from build123d import *

# Parameters (mm, degrees)
ESQUISSE2_W             = 165
ESQUISSE2_H             = 165
BASE_DEPTH              = 30
ESQUISSE3_R             = 15
BLOC_MOTEUR_1_DEPTH     = 80
ESQUISSE4_W             = 10
ESQUISSE4_H             = 22.360679774
ACCES_MOTEUR_DEPTH      = 37
ESQUISSE6_R             = 16.01
BLOC_MOTEUR_2_DEPTH     = 37
ESQUISSE7_R             = 2.5
VIS_MOTEUR_DEPTH        = 121.467838032
ESQUISSE8_R             = 2.5
VIS_PATIN_DEPTH         = 121.467838032
ESQUISSE12_R            = 30
ESPACE_ROUE_DEPTH       = 10
FIXE_PORTE_1_DEPTH      = 2.5
FIXE_PORTE_1_DEPTH_BACK = 10
ESQUISSE14_R            = 2
ESQUISSE15_W            = 5
ESQUISSE15_H            = 10.139320225
FIXE_PORTE_2_DEPTH      = 2.5
ESQUISSE16_R            = 2
FIXE_PORTE_3_DEPTH      = 10
ESQUISSE18_R            = 2
VIDE_CORDE_COTE_DEPTH   = 75
ESQUISSE19_R            = 2
VIDEO_CORDE_HAUT_DEPTH  = 5
CONGE_CORDE_R           = 0.8
ESQUISSE20_R            = 2
BOSS_MAX_PORTE_DEPTH    = 2
ESQUISSE23_W            = 10
ESQUISSE23_H            = 30
VIDE_TIGE_DEPTH         = 10
VIDE_VIS_REACH          = 185.737
ESQUISSE25_R            = 2.5


with BuildPart() as part:
    # Esquisse2 → BASE (new body)
    with BuildSketch(Plane(origin=(0, 0, 0), x_dir=(1, 0, 0), z_dir=(0, 1, 0))):
        Rectangle(ESQUISSE2_W, ESQUISSE2_H)
    extrude(amount=BASE_DEPTH)

    # Esquisse3 → BLOC MOTEUR 1. (cut)
    with BuildSketch(Plane(origin=(82.5, 0, 0), x_dir=(0, 0, -1), z_dir=(1, 0, 0))):
        with Locations((50, 10)):
            Circle(ESQUISSE3_R)
    bloc_moteur_1 = extrude(amount=-BLOC_MOTEUR_1_DEPTH, mode=Mode.SUBTRACT)

    # Esquisse4 → ACCES MOTEUR (cut)
    with BuildSketch(Plane.XZ):
        with Locations((7.5, -50)):
            Rectangle(ESQUISSE4_W, ESQUISSE4_H)
    acces_moteur = extrude(amount=-ACCES_MOTEUR_DEPTH, mode=Mode.SUBTRACT)

    # Esquisse6 → BLOC MOTEUR 2 (cut)
    with BuildSketch(Plane(origin=(82.5, 0, 0), x_dir=(0, 0, -1), z_dir=(1, 0, 0))):
        with Locations((50, 10)):
            Circle(ESQUISSE6_R)
    bloc_moteur_2 = extrude(amount=-BLOC_MOTEUR_2_DEPTH, mode=Mode.SUBTRACT)

    # SYM BLOC MOTEUR: BLOC MOTEUR 1., ACCES MOTEUR, BLOC MOTEUR 2 across plane
    add(bloc_moteur_1.mirror(Plane(origin=(0, 0, 0), x_dir=(0, 0, 1), z_dir=(1, 0, 0))), mode=Mode.SUBTRACT)
    add(acces_moteur.mirror(Plane(origin=(0, 0, 0), x_dir=(0, 0, 1), z_dir=(1, 0, 0))), mode=Mode.SUBTRACT)
    add(bloc_moteur_2.mirror(Plane(origin=(0, 0, 0), x_dir=(0, 0, 1), z_dir=(1, 0, 0))), mode=Mode.SUBTRACT)

    # Esquisse7 → VIS MOTEUR (cut, through all)
    with BuildSketch(Plane.XZ):
        with Locations(Location((-64, -27.497196314, 0), (0, 0, 270))):
            Circle(ESQUISSE7_R)
        with Locations(Location((-24, -28.819660113, 0), (0, 0, 270))):
            Circle(ESQUISSE7_R)
        with Locations(Location((-24, -71.180339887, 0), (0, 0, 270))):
            Circle(ESQUISSE7_R)
        with Locations(Location((-64, -72.502803686, 0), (0, 0, 270))):
            Circle(ESQUISSE7_R)
    vis_moteur = extrude(amount=-VIS_MOTEUR_DEPTH, mode=Mode.SUBTRACT)

    # SYM VIS: VIS MOTEUR across plane
    add(vis_moteur.mirror(Plane(origin=(0, 0, 0), x_dir=(0, 0, 1), z_dir=(1, 0, 0))), mode=Mode.SUBTRACT)

    # Esquisse8 → VIS PATIN (cut, through all)
    with BuildSketch(Plane.XZ):
        with Locations(Location((-52.5, 52.5, 0), (0, 0, 270))):
            Circle(ESQUISSE8_R)
        with Locations(Location((52.5, 52.5, 0), (0, 0, 270))):
            Circle(ESQUISSE8_R)
    extrude(amount=-VIS_PATIN_DEPTH, mode=Mode.SUBTRACT)

    # Esquisse12 → ESPACE ROUE (cut)
    with BuildSketch(Plane.ZY.offset(82.5)):
        with Locations((-50, 10)):
            Circle(ESQUISSE12_R)
    espace_roue = extrude(amount=-ESPACE_ROUE_DEPTH, mode=Mode.SUBTRACT)

    # SYM ESPACE ROUE: ESPACE ROUE across plane
    add(espace_roue.mirror(Plane(origin=(0, 0, 0), x_dir=(0, 0, 1), z_dir=(1, 0, 0))), mode=Mode.SUBTRACT)

    # Esquisse14 → FIXE PORTE 1 (add, two sides: drawn at the far end of the back side and taken through both)
    # profile 1 of 2: a face of its own
    with BuildSketch(Plane(origin=(0, 30, 0), x_dir=(1, 0, 0), z_dir=(0, 1, 0)).offset(-FIXE_PORTE_1_DEPTH_BACK)):
        with BuildLine():
            ThreePointArc((-77.5, 87.245138583), (-80, 89.745138583), (-82.5, 87.245138583))
            Line((-82.5, 87.245138583), (-82.5, 82.5))
            Line((-82.5, 82.5), (-77.5, 82.5))
            Line((-77.5, 82.5), (-77.5, 87.245138583))
        make_face()
        with Locations(Location((-80, 87.245138583, 0), (0, 0, 270))):
            Circle(ESQUISSE14_R, mode=Mode.SUBTRACT)
    # profile 2 of 2: a face of its own
    with BuildSketch(Plane(origin=(0, 30, 0), x_dir=(1, 0, 0), z_dir=(0, 1, 0)).offset(-FIXE_PORTE_1_DEPTH_BACK)):
        with BuildLine():
            Line((77.5, 87.245138583), (77.5, 82.5))
            Line((77.5, 82.5), (82.5, 82.5))
            Line((82.5, 82.5), (82.5, 87.245138583))
            ThreePointArc((82.5, 87.245138583), (80, 89.745138583), (77.5, 87.245138583))
        make_face()
        with Locations(Location((80, 87.245138583, 0), (0, 0, 270))):
            Circle(ESQUISSE14_R, mode=Mode.SUBTRACT)
    extrude(amount=FIXE_PORTE_1_DEPTH + FIXE_PORTE_1_DEPTH_BACK)

    # Esquisse15 → FIXE PORTE 2 (add)
    with BuildSketch(Plane(origin=(0, 30, 0), x_dir=(1, 0, 0), z_dir=(0, 1, 0))):
        with Locations((-80, 77.430339887)):
            Rectangle(ESQUISSE15_W, ESQUISSE15_H)
        with Locations((80, 77.430339887)):
            Rectangle(ESQUISSE15_W, ESQUISSE15_H)
    extrude(amount=FIXE_PORTE_2_DEPTH)

    # Esquisse16 → FIXE PORTE 3 (add)
    # profile 1 of 2: a face of its own
    with BuildSketch(Plane.XZ):
        with BuildLine():
            Line((-82.5, -82.5), (-82.5, -87.245138583))
            ThreePointArc((-82.5, -87.245138583), (-80, -89.745138583), (-77.5, -87.245138583))
            Line((-77.5, -87.245138583), (-77.5, -82.5))
            Line((-77.5, -82.5), (-82.5, -82.5))
        make_face()
        with Locations(Location((-80, -87.245138583, 0), (0, 0, 90))):
            Circle(ESQUISSE16_R, mode=Mode.SUBTRACT)
    # profile 2 of 2: a face of its own
    with BuildSketch(Plane.XZ):
        with BuildLine():
            Line((82.5, -82.5), (77.5, -82.5))
            Line((77.5, -82.5), (77.5, -87.245138583))
            ThreePointArc((77.5, -87.245138583), (80, -89.745138583), (82.5, -87.245138583))
            Line((82.5, -87.245138583), (82.5, -82.5))
        make_face()
        with Locations(Location((80, -87.245138583, 0), (0, 0, 90))):
            Circle(ESQUISSE16_R, mode=Mode.SUBTRACT)
    extrude(amount=-FIXE_PORTE_3_DEPTH)

    # Esquisse18 → VIDE CORDE COTE (cut)
    with BuildSketch(Plane(origin=(82.5, 0, 0), x_dir=(0, 0, -1), z_dir=(1, 0, 0))):
        with Locations((79.5, 27)):
            Circle(ESQUISSE18_R)
    vide_corde_cote = extrude(amount=-VIDE_CORDE_COTE_DEPTH, mode=Mode.SUBTRACT)

    # Esquisse19 → VIDEO CORDE HAUT (cut)
    with BuildSketch(Plane(origin=(0, 30, 0), x_dir=(1, 0, 0), z_dir=(0, 1, 0))):
        with Locations(Location((9.5, 79.5, 0), (0, 0, 270))):
            Circle(ESQUISSE19_R)
    video_corde_haut = extrude(amount=-VIDEO_CORDE_HAUT_DEPTH, mode=Mode.SUBTRACT)

    # SYM CORDE: VIDE CORDE COTE, VIDEO CORDE HAUT across plane
    add(vide_corde_cote.mirror(Plane(origin=(0, 0, 0), x_dir=(0, 0, 1), z_dir=(1, 0, 0))), mode=Mode.SUBTRACT)
    add(video_corde_haut.mirror(Plane(origin=(0, 0, 0), x_dir=(0, 0, 1), z_dir=(1, 0, 0))), mode=Mode.SUBTRACT)

    # CONGE CORDE
    conge_corde_edges = [part.edges().sort_by_distance(p)[0] for p in [
        (9.5, 30, -81.5),
        (-9.5, 30, -81.5),
    ]]
    fillet(conge_corde_edges, radius=CONGE_CORDE_R)

    # Esquisse20 → BOSS MAX PORTE (add)
    with BuildSketch(Plane(origin=(82.5, 0, 0), x_dir=(0, 0, -1), z_dir=(1, 0, 0))):
        with BuildLine():
            Line((72.360679775, 30), (72.360679775, 32.5))
            Line((72.360679775, 32.5), (87.360679775, 32.5))
            Line((87.360679775, 32.5), (87.360679775, 0))
            Line((87.360679775, 0), (78.284271247, 0))
            ThreePointArc((78.284271247, 0), (79.431747587, 15.811388301), (72.360679775, 30))
        make_face()
        with Locations((79.5, 27)):
            Circle(ESQUISSE20_R, mode=Mode.SUBTRACT)
    boss_max_porte = extrude(amount=BOSS_MAX_PORTE_DEPTH)

    # SYM MAX PORTE: BOSS MAX PORTE across plane
    add(boss_max_porte.mirror(Plane(origin=(0, 0, 0), x_dir=(0, 0, 1), z_dir=(1, 0, 0))))

    # Esquisse23 → VIDE TIGE (cut)
    with BuildSketch(Plane(origin=(82.5, 0, 0), x_dir=(0, 0, -1), z_dir=(1, 0, 0))):
        with Locations((-72.5, 15)):
            Rectangle(ESQUISSE23_W, ESQUISSE23_H)
        with Locations((7.5, 15)):
            Rectangle(ESQUISSE23_W, ESQUISSE23_H)
    vide_tige = extrude(amount=-VIDE_TIGE_DEPTH, mode=Mode.SUBTRACT)

    # SYM TIGE: VIDE TIGE across plane
    add(vide_tige.mirror(Plane(origin=(0, 0, 0), x_dir=(0, 0, 1), z_dir=(1, 0, 0))), mode=Mode.SUBTRACT)

    # Esquisse25 → VIDE VIS (cut, up to next)
    with BuildSketch(Plane(origin=(72.5, 0, 0), x_dir=(0, 0, -1), z_dir=(1, 0, 0)), mode=Mode.PRIVATE) as vide_vis_sk1:
        with Locations((-72.5, 25)):
            Circle(ESQUISSE25_R)
    vide_vis_tool1 = extrude(vide_vis_sk1.sketch, amount=-VIDE_VIS_REACH, mode=Mode.PRIVATE) & part.part
    # Esquisse25 → VIDE VIS (cut, up to next)
    with BuildSketch(Plane(origin=(72.5, 0, 0), x_dir=(0, 0, -1), z_dir=(1, 0, 0)), mode=Mode.PRIVATE) as vide_vis_sk2:
        with Locations((-72.5, 15)):
            Circle(ESQUISSE25_R)
    vide_vis_tool2 = extrude(vide_vis_sk2.sketch, amount=-VIDE_VIS_REACH, mode=Mode.PRIVATE) & part.part
    # Esquisse25 → VIDE VIS (cut, up to next)
    with BuildSketch(Plane(origin=(72.5, 0, 0), x_dir=(0, 0, -1), z_dir=(1, 0, 0)), mode=Mode.PRIVATE) as vide_vis_sk3:
        with Locations((-72.5, 5)):
            Circle(ESQUISSE25_R)
    vide_vis_tool3 = extrude(vide_vis_sk3.sketch, amount=-VIDE_VIS_REACH, mode=Mode.PRIVATE) & part.part
    # Esquisse25 → VIDE VIS (cut, up to next)
    with BuildSketch(Plane(origin=(72.5, 0, 0), x_dir=(0, 0, -1), z_dir=(1, 0, 0)), mode=Mode.PRIVATE) as vide_vis_sk4:
        with Locations(Location((7.5, 5, 0), (0, 0, 180))):
            Circle(ESQUISSE25_R)
    vide_vis_tool4 = extrude(vide_vis_sk4.sketch, amount=-VIDE_VIS_REACH, mode=Mode.PRIVATE) & part.part
    # Esquisse25 → VIDE VIS (cut, up to next)
    with BuildSketch(Plane(origin=(72.5, 0, 0), x_dir=(0, 0, -1), z_dir=(1, 0, 0)), mode=Mode.PRIVATE) as vide_vis_sk5:
        with Locations(Location((7.5, 25, 0), (0, 0, 180))):
            Circle(ESQUISSE25_R)
    vide_vis_tool5 = extrude(vide_vis_sk5.sketch, amount=-VIDE_VIS_REACH, mode=Mode.PRIVATE) & part.part
    # Esquisse25 → VIDE VIS (cut, up to next)
    with BuildSketch(Plane(origin=(72.5, 0, 0), x_dir=(0, 0, -1), z_dir=(1, 0, 0)), mode=Mode.PRIVATE) as vide_vis_sk6:
        with Locations(Location((7.5, 15, 0), (0, 0, 180))):
            Circle(ESQUISSE25_R)
    vide_vis_tool6 = extrude(vide_vis_sk6.sketch, amount=-VIDE_VIS_REACH, mode=Mode.PRIVATE) & part.part
    add(vide_vis_tool1.solids().sort_by_distance((72.5, 25, 72.5))[0], mode=Mode.SUBTRACT)
    add(vide_vis_tool2.solids().sort_by_distance((72.5, 15, 72.5))[0], mode=Mode.SUBTRACT)
    add(vide_vis_tool3.solids().sort_by_distance((72.5, 5, 72.5))[0], mode=Mode.SUBTRACT)
    add(vide_vis_tool4.solids().sort_by_distance((72.5, 5, -7.5))[0], mode=Mode.SUBTRACT)
    add(vide_vis_tool5.solids().sort_by_distance((72.5, 25, -7.5))[0], mode=Mode.SUBTRACT)
    add(vide_vis_tool6.solids().sort_by_distance((72.5, 15, -7.5))[0], mode=Mode.SUBTRACT)


solid = part.part
Check sheet for the modelled part. Datum: model origin and axes. Units: mm. A direction names the side the tool comes from. Coordinates: 2 decimals unless noted, no trailing zeros. Write each loop counter-clockwise with the first axis right and the second up, starting at its lowest first coordinate (ties: lowest second). Pieces come first, ordered by that corner, then holes. Notation, with made-up numbers: M 36.25,4.5 L 72.25,4.5 A13 cw 72.25,12.5 Z; hole C -12.5,-5 d11. An arc over 180 degrees is marked long. Answer as CSV lines item,"result".
Q1. Mould release check, pull along Y, two halves, no side actions. Record for faces 5 (the face through (81, 32.5, -79)), 6 (the face through (-24, 25, -50)), 7 (the face through (84.5, 16, -82)): released by +Y, released by -Y, zero draft, split by the parting line, or undercut.
Check result:
face 5,"released by +Y"
face 6,"undercut"
face 7,"zero draft"
Q2. Set-up check for faces 1 (the face through (-10, 25, -80)), 2 (the face through (-82.5, 15, 33)), 3 (the face through (12.5, 26, -50)), 4 (the face through (77.5, 5, -85)): record each of +Z, -Z, +X, -X, +Y, -Y from which the full face is reachable in a straight line by a thin tool's end or side.
Check result:
face 1,"+Y"
face 2,"+Z, -X, +Y, -Y"
face 3,"+Y, -Y"
face 4,"-Z, +Y, -Y"
Q3. Material ranges on probe 1 along X at (y, z) = (10, 54); probe 2 along Z at (x, y) = (63.5, 16.5); probe 3 along Z at (x, y) = (-52, 13), recorded low to high. Write a range as from..to.
Check result:
probe 1,"-82.5..-54.5, -50.5..50.5, 54.5..82.5"
probe 2,"-82.5..-74.95, -70.05..-64.63, -35.37..-29.95, -25.05..-9.5, -5.5..70.5, 74.5..82.5"
probe 3,"-82.5..-65.73, -34.27..-9, -6..50.05, 54.95..71, 74..82.5"
Q4. Cross-section at A-A (x = 24). Count the separate pieces of the cut face and the enclosed holes in it, then the cut area to 3 significant figures.
Check result:
separate pieces,"3"
enclosed holes,"7"
area,"3,890 mm^2"
Q5. Go/stop test with flat-tipped pins: pin 1 (3 mm diameter, centred on x = 75, y = 8, fed in from -Z); pin 2 (4.5 mm diameter, centred on y = 15, z = -7.5, fed in from +X); pin 3 (5 mm diameter, centred on x = 56.5, z = -55, fed in from -Y); pin 4 (1.5 mm diameter, centred on y = 12.5, z = -5, fed in from -X). Record where each tip stops, or that it passes through.
Check result:
pin 1,"z = -82.5"
pin 2,"through"
pin 3,"y = 24.14"
pin 4,"x = -72.5"
Q6. Cross-section at B-B (z = -7.5). Record the boundary of the cut face in (x, y), then the cut area to 4 significant figures.
Check result:
outline,"M -72.5,0 L 72.5,0 L 72.5,2.5 L -72.5,2.5 Z; M -72.5,7.5 L 72.5,7.5 L 72.5,12.5 L -72.5,12.5 Z; M -72.5,17.5 L 72.5,17.5 L 72.5,22.5 L -72.5,22.5 Z; M -72.5,27.5 L 72.5,27.5 L 72.5,30 L -72.5,30 Z"
area,"2,175 mm^2"
